Verification items for this drawing (mm, ordinates from the low corner). Round coordinates to 2 decimals unless told otherwise and drop trailing zeros. Order: outer loops, then holes, each group sorted by start corner. A loop starts at its lowest first (then second) coordinate and runs counter-clockwise, first axis right, second up. Notation, with made-up numbers: M -23,72.5 L 30,72.5 A18 ccw 30,103.5 Z; hole C -8,-22.75 d2. An arc over 180 degrees is marked long. Use CSV: the item, a comma, the result in double quotes. Start each with the question number.
Q1. Scan lines: line 1 (Z direction, x = 11, y = 11); line 2 (Z direction, x = 50, y = 4.25); line 3 (X direction, y = 5, z = 13.5). Record each from-to range of solid material in increasing order.
Q2. Sectioned sample at B-B (y = 8). Enter the section's corners in (x, z), and give its area (3 significant figures).
Q3. Sectioned sample at A-A (z = 12). Enter the section's corners in (x, y), and give its area (3 significant figures).
Q4. Mould release check, pull along X, two halves, no side actions. Record for the marked faces 1, 2 and 3: +X half, -X half, draft (parallel to the pull), parting line (faces both ways), or undercut.
Q5. Sectioned sample at D-D (x = 50). Enter the section's corners in (y, z), and give its area (3 significant figures).
Q6. Sectioned sample at C-C (z = 50). Enter the section's corners in (x, y).
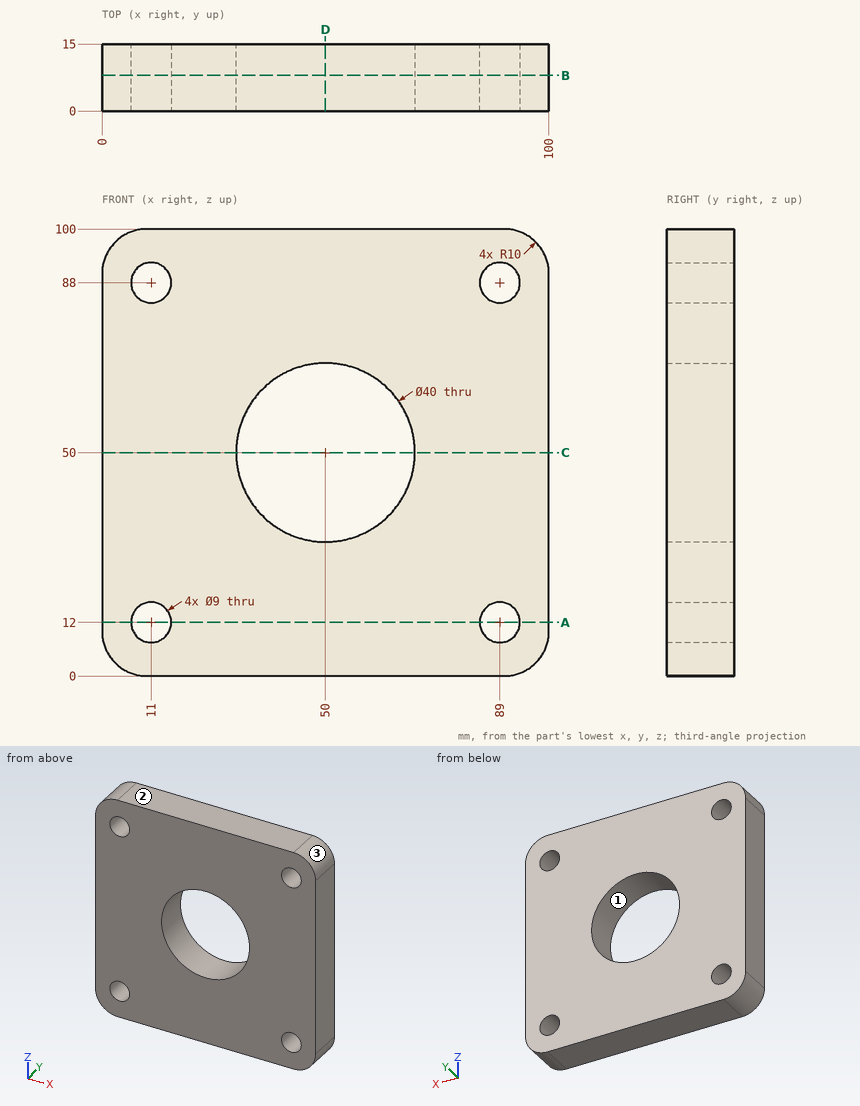
Verdict:
1,line 1,"z = 0 to 7.5, 16.5 to 83.5, 92.5 to 100"
1,line 2,"z = 0 to 30, 70 to 100"
1,line 3,"x = 0 to 6.76, 15.24 to 84.76, 93.24 to 100"
2,outline,"M 0,10 A10 ccw 10,0 L 90,0 A10 ccw 100,10 L 100,90 A10 ccw 90,100 L 10,100 A10 ccw 0,90 Z; hole C 11,12 d9; hole C 11,88 d9; hole C 50,50 d40; hole C 89,12 d9; hole C 89,88 d9"
2,area,"8,400 mm²"
3,outline,"M 0,0 L 6.5,0 L 6.5,15 L 0,15 Z; M 15.5,0 L 84.5,0 L 84.5,15 L 15.5,15 Z; M 93.5,0 L 100,0 L 100,15 L 93.5,15 Z"
3,area,"1,230 mm²"
4,face 1,"undercut"
4,face 2,"draft"
4,face 3,"+X half"
5,outline,"M 0,0 L 15,0 L 15,30 L 0,30 Z; M 0,70 L 15,70 L 15,100 L 0,100 Z"
5,area,"900 mm²"
6,outline,"M 0,0 L 30,0 L 30,15 L 0,15 Z; M 70,0 L 100,0 L 100,15 L 70,15 Z"
